Work out the finished part from the listing and answer in its coordinate system (mm). A direction names the side the tool comes from. Coordinates: 2 decimals unless noted, no trailing zeros. Order: outer loops, then holes, each group sorted by start corner. A loop starts at its lowest first (then second) coordinate and runs counter-clockwise, first axis right, second up. Notation, with made-up numbers: (74, 6.25) -> (105, 6.25) arc R38 ccw to (105, 45.25) -> close; hole circle Ø1 at (16.5, 81.25). An arc over 180 degrees is marked (long way). Use one line per item in the form item = value.
from build123d import *

# Parameters (mm, degrees)
BOSS_EXTRUDE1_DEPTH = 20.32
SKETCH2_W           = 10.166490401
SKETCH2_H           = 81.316938585
SKETCH2_W_2         = 10.166490402
SKETCH2_H_2         = 81.316938584
SKETCH2_W_3         = 82.271298803
SKETCH2_H_3         = 10.16
CUT_EXTRUDE2_DEPTH  = 137.414
CUT_EXTRUDE3_DEPTH  = 21.3200001
SKETCH5_W           = 82.296
SKETCH5_H           = 10.16
CUT_EXTRUDE4_DEPTH  = 21.3200001
CUT_EXTRUDE5_DEPTH  = 21.3200001


with BuildPart() as part:
    # Sketch1 → Boss-Extrude1 (new body)
    with BuildSketch(Plane.XY):
        with BuildLine():
            Line((0, 0), (1345.447057269, 0))
            Line((1345.447057269, 0), (1156.937235756, -454.288839135))
            add(Edge.make_bspline(
                [(1156.937235756, -454.288839135), (1155.965204773, -456.631331547), (1154.630956054, -458.816896883), (1152.225947859, -461.69350105), (1151.355065983, -462.590813772), (1149.473312624, -464.260936999), (1148.45987476, -465.033112958), (1146.360299176, -466.401155283), (1145.26635201, -467.004685932), (1142.990856866, -468.052074807), (1141.798989191, -468.498505895), (1138.174492983, -469.560599459), (1135.699262078, -469.911644948), (1133.16419506, -469.9)],
                knots=[0, 0, 0, 0, 0.25, 0.25, 0.375, 0.375, 0.5, 0.5, 0.625, 0.625, 0.75, 0.75, 1, 1, 1, 1], degree=3))
            Line((1133.16419506, -469.9), (212.282862208, -469.9))
            add(Edge.make_bspline(
                [(188.509821513, -454.288839135), (189.481852496, -456.631331547), (190.816101215, -458.816896883), (193.22110941, -461.69350105), (194.091991286, -462.590813772), (195.973744645, -464.260936999), (196.987182509, -465.033112958), (199.086758093, -466.401155283), (200.180705259, -467.004685932), (202.456200403, -468.052074807), (203.648068078, -468.498505895), (207.272564286, -469.560599459), (209.747795191, -469.911644948), (212.282862208, -469.9)],
                knots=[0, 0, 0, 0, 0.25, 0.25, 0.375, 0.375, 0.5, 0.5, 0.625, 0.625, 0.75, 0.75, 1, 1, 1, 1], degree=3))
            Line((188.509821513, -454.288839135), (0, 0))
        make_face()
    extrude(amount=BOSS_EXTRUDE1_DEPTH)

    # Sketch2 → Cut-Extrude2 (cut)
    with BuildSketch(Plane.XY.offset(20.32)):
        with Locations((461.924984631, -337.764592123)):
            Rectangle(SKETCH2_W, SKETCH2_H)
        with Locations((883.522072638, -337.764592123)):
            Rectangle(SKETCH2_W_2, SKETCH2_H)
        with Locations((883.522072638, -175.130714953)):
            Rectangle(SKETCH2_W_2, SKETCH2_H_2)
        with Locations((461.924984631, -175.130714953)):
            Rectangle(SKETCH2_W, SKETCH2_H_2)
        with Locations((837.303178036, -464.82)):
            Rectangle(SKETCH2_W_3, SKETCH2_H_3)
        with Locations((672.723528635, -464.82)):
            Rectangle(SKETCH2_W_3, SKETCH2_H_3)
        with Locations((508.143879233, -464.82)):
            Rectangle(SKETCH2_W_3, SKETCH2_H_3)
    extrude(amount=-CUT_EXTRUDE2_DEPTH, mode=Mode.SUBTRACT)

    # Sketch4 → Cut-Extrude3 (cut, through all)
    with BuildSketch(Plane.XY.offset(20.32)):
        Polygon((0, 0), (1345.447057269, 0), (1327.002268746, -44.45), (18.444788523, -44.45), align=None)
    extrude(amount=-CUT_EXTRUDE3_DEPTH, mode=Mode.SUBTRACT)

    # Sketch5 → Cut-Extrude4 (cut, through all)
    with BuildSketch(Plane.XY.offset(20.32)):
        with Locations((508.131528634, -49.53)):
            Rectangle(SKETCH5_W, SKETCH5_H)
        with Locations((672.723528634, -49.53)):
            Rectangle(SKETCH5_W, SKETCH5_H)
        with Locations((837.315528634, -49.53)):
            Rectangle(SKETCH5_W, SKETCH5_H)
    extrude(amount=-CUT_EXTRUDE4_DEPTH, mode=Mode.SUBTRACT)

    # Sketch6 → Cut-Extrude5 (cut, through all)
    with BuildSketch(Plane.XY.offset(20.32)):
        Polygon((192.807539001, -448.077869782), (224.982862208, -469.9), (232.080223429, -549.766419732), (-59.510742861, -242.335130221), (-120.238907144, 37.382474964), (56.544788523, -44.45), (56.544788523, -119.698975594), align=None)
        Polygon((1120.46419506, -469.9), (1113.36683384, -549.766419732), (1404.95780013, -242.335130221), (1465.685964413, 37.382474964), (1288.902268746, -44.45), (1288.902268746, -119.698975594), (1152.639518267, -448.077869782), align=None)
    extrude(amount=-CUT_EXTRUDE5_DEPTH, mode=Mode.SUBTRACT)


solid = part.part
(1) Which of the six approach directions +Z, -Z, +X, -X, +Y, -Y give full straight-line access (tool end or side, diameter ignored) to faces 1 (the flat face through (672, -54.61, 10)), 2 (the flat face through (888.605, -176, 10)), 3 (the flat face through (672, -459.74, 10))?
Data:
face_1 = +Z, -Z, +Y
face_2 = +Z, -Z
face_3 = +Z, -Z, -Y
(2) Section B-B on x = 853.5 is taken. Write down the section's boundary in (y, z).
Data:
outline = (-459.74, 0) -> (-54.61, 0) -> (-54.61, 20.32) -> (-459.74, 20.32) -> close
(3) Section D-D on x = 179.5 is taken. Write down the section's boundary in (y, z).
Data:
outline = (-416.01, 0) -> (-44.45, 0) -> (-44.45, 20.32) -> (-416.01, 20.32) -> close
(4) Section A-A on y = -319 is taken. Write down the section's boundary in (x, z), plus the area to 3 significant figures.
Data:
outline = (139.25, 0) -> (456.84, 0) -> (456.84, 20.32) -> (139.25, 20.32) -> close; (467.01, 0) -> (878.44, 0) -> (878.44, 20.32) -> (467.01, 20.32) -> close; (888.61, 0) -> (1206.2, 0) -> (1206.2, 20.32) -> (888.61, 20.32) -> close
area = 21,300 mm²
(5) Each of these flat-tipped pins is pushed along its axis until it touches: P1, Ø10, axis at y = -159.5, z = 8.5, coming from the -X side; P2, Ø4, axis at y = -379.5, z = 15.5, coming from the -X side; P3, Ø3, axis at y = -349.5, z = 7, coming from the +X side; P4, Ø3, axis at x = 250, y = -325.5, coming from the -Z side. Where does it stop, or does it pass through?
Data:
P1 = 70.99
P2 = 163.52
P3 = 1194.17
P4 = 0
(6) The mould has two halves that part along X. Classify faces 4 (the flat face through (208.67, -458.836, 10.302)), 5 (the flat face through (265, -44.45, 10)), 6 (the flat face through (467.008, -338, 10)): released by +X, released by -X, zero draft, split by the parting line, or undercut.
Data:
face_4 = released by -X
face_5 = zero draft
face_6 = undercut
(7) Section C-C on z = 6 is taken. Count the separate pieces of the cut face and the enclosed holes in it, plus the area to 3 significant figures.
Data:
separate_pieces = 1
enclosed_holes = 4
area = 465,000 mm²
(8) Straight lines are drawn through the part: line 1 along Y through (x, z) = (477, 10.5); line 2 along X through (y, z) = (-340.5, 10.5); line 3 along X through (y, z) = (-153.5, 5.5). For each, find the intervals that lie inside material, in ascending order.
Data:
line_1 = -459.74 to -54.61
line_2 = 148.17 to 456.84, 467.01 to 878.44, 888.61 to 1197.28
line_3 = 70.57 to 456.84, 467.01 to 878.44, 888.61 to 1274.88
